from build123d import *

# Parameters (mm, degrees)
F1_DEPTH = 25
F2_R     = 5
F3_T     = -2.5


with BuildPart() as f1:
    # F0 (on Top) → F1 (new body)
    with BuildSketch(Plane.XY):
        Polygon((19.44085, -15.114036), (23.937801, 5.776022), (10.409099, 22.316617), (-10.957867, 22.052344), (-24.073335, 5.182207), (-19.061091, -15.590238), (0.304543, -24.622916), align=None)
    extrude(amount=F1_DEPTH)

    # F2
    f2_edges = [f1.edges().sort_by_distance(p)[0] for p in [
        (21.689326, -4.669007, 0),
        (17.17345, 14.046319, 0),
        (-0.274384, 22.184481, 0),
        (-17.515601, 13.617276, 0),
        (-21.567213, -5.204016, 0),
        (-9.378274, -20.106577, 0),
        (9.872697, -19.868476, 0),
    ]]
    fillet(f2_edges, radius=F2_R)

    # F3
    f3_openings = [f1.faces().sort_by_distance(p)[0] for p in [
        (0, 0, 25),
    ]]
    offset(amount=F3_T, openings=f3_openings)


solid = f1.part
Check sheet for the modelled part. Datum: model origin and axes. Units: mm. A direction names the side the tool comes from. Give positions to 0.01 mm unless a question says otherwise; leave off trailing zeros. Write each loop counter-clockwise with the first axis right and the second up, starting at its lowest first coordinate (ties: lowest second). Pieces come first, ordered by that corner, then holes. Notation, with made-up numbers: (-37.75, 18.5) -> (11.25, 18.5) arc R22 ccw to (11.25, 35.5) -> close; hole circle Ø11 at (59, 20). An arc over 180 degrees is marked (long way). Use one line per item in the form item = value. Start each with the question number.
1. Thickness scan on line 1 along Z through (x, y) = (-3.5, 9); line 2 along Y through (x, z) = (-3.5, 18.5); line 3 along X through (y, z) = (9.5, 11). Record the ranges inside material, lowest first. Write a range as from..to.
2. Access from +Z, -Z, +X, -X, +Y, -Y to the whole of each face (thin tool, end or side, straight path). Record for faces 1 (the cylindrical face through (-0.406, 20.757, 1.504)), 2 (the flat face through (0, -1, 0)), 3 (the flat face through (19.217, -4.273, 14.86)).
3. Mould release check, pull along Y, two halves, no side actions. Record for faces 4 (the flat face through (0, 20, 25)), 5 (the flat face through (-17.42, 13.74, 14.86)), 6 (the cylindrical face through (9.372, -18.525, 1.504)), 7 (the flat face through (-8.442, -17.785, 14.86)): pulls with the +Y half, pulls with the -Y half, needs draft (parallel to the pull), parting line crosses it, or undercut.
4. Section check A-A (z = 21). Record the cut outline in (x, y), and give its area (3 significant figures).
5. Go/stop test with flat-tipped pins: P1, Ø12, axis at y = -0.5, z = 10.5, coming from the -X side; P2, Ø3, axis at y = -19, z = 21, coming from the -X side; P3, Ø2, axis at x = -7, y = -3.5, coming from the +Z side. Record where each tip stops, or that it passes through.
Conclusion:
q1.line_1 = 0..2.5
q1.line_2 = -22.85..-20.09, 19.64..22.14
q1.line_3 = -20.72..-17.55, 17.66..20.89
q2.face_1 = -Z, -X, +Y
q2.face_2 = -Z, +X, -X, +Y, -Y
q2.face_3 = +Z
q3.face_4 = needs draft
q3.face_5 = pulls with the +Y half
q3.face_6 = pulls with the -Y half
q3.face_7 = undercut
q4.outline = (-24.07, 5.18) -> (-19.06, -15.59) -> (0.3, -24.62) -> (19.44, -15.11) -> (23.94, 5.78) -> (10.41, 22.32) -> (-10.96, 22.05) -> close; hole (-21.36, 4.6) -> (-16.91, -13.83) -> (0.27, -21.85) -> (17.25, -13.41) -> (21.24, 5.13) -> (9.24, 19.8) -> (-9.72, 19.57) -> close
q4.area = 353 mm²
q5.P1 = -24.07
q5.P2 = -14.97
q5.P3 = 2.5
